from build123d import *

# Parameters (mm, degrees)
BOSS_EXTRUDE1_DEPTH = 50.8
CHAMFER2_SIZE       = 17.78
CHAMFER3_SIZE       = 17.78
SKETCH8_W           = 2.032
SKETCH8_H           = 149.939355631
CUT_EXTRUDE3_DEPTH  = 6.35


with BuildPart() as part:
    # Sketch6 → Boss-Extrude1 (new body)
    with BuildSketch(Plane.XY):
        Polygon((0, 0), (0, 76.2), (228.6, 76.2), (228.6, 127), (355.6, 127), (254, 0), align=None)
    extrude(amount=BOSS_EXTRUDE1_DEPTH)

    # Chamfer2
    chamfer2_edges = [part.edges().sort_by_distance(p)[0] for p in [
        (304.8, 63.5, 50.8),
    ]]
    chamfer(chamfer2_edges, length=CHAMFER2_SIZE)

    # Chamfer3
    chamfer3_edges = [part.edges().sort_by_distance(p)[0] for p in [
        (304.8, 63.5, 0),
    ]]
    chamfer(chamfer3_edges, length=CHAMFER3_SIZE)

    # Sketch8 → Cut-Extrude3 (cut)
    with BuildSketch(Plane(origin=(154.87804878, -123.902439024, 0), x_dir=(0, 0, -1), z_dir=(0.7808688094430302, -0.6246950475544245, 0))):
        with Locations((-25.4, 239.992219895)):
            Rectangle(SKETCH8_W, SKETCH8_H)
    extrude(amount=-CUT_EXTRUDE3_DEPTH, mode=Mode.SUBTRACT)


solid = part.part
Could you check a few things on this model? Use its own coordinates, in mm. A direction names the side the tool comes from. Coordinates: 2 decimals unless noted, no trailing zeros. Write each loop counter-clockwise with the first axis right and the second up, starting at its lowest first coordinate (ties: lowest second). Pieces come first, ordered by that corner, then holes. Notation, with made-up numbers: (-19, -16.5) - (13, -16.5) arc R10 ccw to (13, -10.5) - close; hole circle Ø7 at (-34.5, -9). An arc over 180 degrees is marked (long way). Put each result on its own line as item: value. Start each with the question number.
Q1. I want a section at C-C on x = 83. Write out the boundary of the cut face in (y, z).
Q2. I want a section at A-A on y = 92.5. Write out the boundary of the cut face in (x, z), plus the area to 3 significant figures.
Q3. Which directions (+Z, -Z, +X, -X, +Y, -Y) give clear straight access to the entire face, cutting with the end or side of a thin tool? Please do faces 4 (the flat face through (0, 38, 25)), 5 (the flat face through (228.6, 101, 25)).
Q4. Thinking about a two-plate mould opening in Z: for faces 1 (the flat face through (302, 65, 24.384)), 2 (the flat face through (294.1, 64.5, 42)), 3 (the flat face through (113, 76.2, 25)), which applies, pulls with the +Z half, pulls with the -Z half, needs draft (parallel to the pull), parting line crosses it, or undercut?
Q5. Please list where these lines run through material, in increasing order: L1, parallel to Y at x = 54.5, z = 14; L2, parallel to Y at x = 282, z = 16; L3, parallel to X at y = 35.5, z = 19.
Q6. I want a section at D-D on y = 40.5. Write out the boundary of the cut face in (x, z).
Q7. I want a section at B-B on z = 13. Write out the boundary of the cut face in (x, y).
Q8. I'm going to push flat-ended pins straight in: P1, Ø1, axis at y = 112, z = 37, coming from the +X side; P2, Ø3, axis at y = 101.5, z = 29.5, coming from the +X side; P3, Ø4, axis at x = 86, z = 40, coming from the +Y side. Where does each tip first touch, or does it pass through?
Checks:
1. outline: (0, 0) - (76.2, 0) - (76.2, 50.8) - (0, 50.8) - close
2. outline: (228.6, 0) - (305.23, 0) - (328, 17.78) - (328, 24.38) - (319.87, 24.38) - (319.87, 26.42) - (328, 26.42) - (328, 33.02) - (305.23, 50.8) - (228.6, 50.8) - close
2. area: 4,630 mm²
3. face 4: +Z, -Z, -X, +Y, -Y
3. face 5: +Z, -Z, -X, +Y
4. face 1: undercut
4. face 2: pulls with the +Z half
4. face 3: needs draft
5. L1: 0 to 76.2
5. L2: 37.85 to 127
5. L3: 0 to 282.4
6. outline: (0, 0) - (263.63, 0) - (286.4, 17.78) - (286.4, 24.38) - (278.27, 24.38) - (278.27, 26.42) - (286.4, 26.42) - (286.4, 33.02) - (263.63, 50.8) - (0, 50.8) - close
7. outline: (0, 0) - (247.88, 0) - (349.48, 127) - (228.6, 127) - (228.6, 76.2) - (0, 76.2) - close
8. P1: x = 339.26
8. P2: x = 336.4
8. P3: y = 76.2
